Input: part model. Units: mm. Frame: model coordinates. A direction names the side the tool comes from. Coordinates: 2 decimals unless noted, no trailing zeros. Order: outer loops, then holes, each group sorted by start corner. A loop starts at its lowest first (then second) coordinate and runs counter-clockwise, first axis right, second up. Notation, with made-up numbers: (-22.5, 44.25) - (22.5, 44.25) arc R19 ccw to (22.5, 72.25) - close; hole circle Ø3 at (53.25, 61). An arc over 180 degrees is marked (long way). One line per question, with ' | ' between items.
from build123d import *

# Parameters (mm, degrees)
SKETCH1_R           = 2.75
SKETCH1_R_2         = 1.75
SKETCH1_W           = 5.5
SKETCH1_H           = 5.5
BOSS_EXTRUDE1_DEPTH = 1
SKETCH2_R           = 2.75
SKETCH2_R_2         = 1.75
BOSS_EXTRUDE2_DEPTH = 2.8
SKETCH3_W           = 25.5
SKETCH3_H           = 35.5
CUT_EXTRUDE1_DEPTH  = 2.8


with BuildPart() as part:
    # Sketch1 → Boss-Extrude1 (new body)
    # profile 1 of 11: a face of its own
    with BuildSketch(Plane(origin=(0, 0, 0), x_dir=(1, 0, 0), z_dir=(0, 1, 0))):
        with Locations((-15, -15)):
            Circle(SKETCH1_R)
        with Locations(Location((-15, -15, 0), (0, 0, 270))):
            Circle(SKETCH1_R_2, mode=Mode.SUBTRACT)
    # profile 2 of 11: a face of its own
    with BuildSketch(Plane(origin=(0, 0, 0), x_dir=(1, 0, 0), z_dir=(0, 1, 0))):
        with BuildLine():
            add(Edge.make_bspline(
                [(0, -7.5), (-1.590584075, -5.319747163), (-2.75, -2.75)],
                knots=[0.745921805, 0.745921805, 0.745921805, 1, 1, 1], degree=2))
            add(Edge.make_bspline(
                [(-15, -12.25), (-5.706246464, -10.868692238), (-2.75, -2.75)],
                knots=[0, 0, 0, 1, 1, 1], degree=2))
            ThreePointArc((-15, -12.25), (-13.055456352, -13.055456352), (-12.25, -15))
            ThreePointArc((-12.25, -15), (-12.459331286, -16.052379439), (-13.055456352, -16.944543648))
            add(Edge.make_bspline(
                [(-13.055456352, -16.944543648), (-4.669630712, -13.900778032), (0, -7.5)],
                knots=[0, 0, 0, 0.745921805, 0.745921805, 0.745921805], degree=2))
        make_face()
    # profile 3 of 11: a face of its own
    with BuildSketch(Plane(origin=(0, 0, 0), x_dir=(1, 0, 0), z_dir=(0, 1, 0))):
        with BuildLine():
            add(Edge.make_bspline(
                [(0, -7.5), (1.590584075, -5.319747163), (2.75, -2.75)],
                knots=[0.745921805, 0.745921805, 0.745921805, 1, 1, 1], degree=2))
            Line((2.75, -2.75), (-2.75, -2.75))
            add(Edge.make_bspline(
                [(0, -7.5), (-1.590584075, -5.319747163), (-2.75, -2.75)],
                knots=[0.745921805, 0.745921805, 0.745921805, 1, 1, 1], degree=2))
        make_face()
    # profile 4 of 11: a face of its own
    with BuildSketch(Plane(origin=(0, 0, 0), x_dir=(1, 0, 0), z_dir=(0, 1, 0))):
        Rectangle(SKETCH1_W, SKETCH1_H)
    # profile 5 of 11: a face of its own
    with BuildSketch(Plane(origin=(0, 0, 0), x_dir=(1, 0, 0), z_dir=(0, 1, 0))):
        with BuildLine():
            add(Edge.make_bspline(
                [(15, -12.25), (5.706246464, -10.868692238), (2.75, -2.75)],
                knots=[0, 0, 0, 1, 1, 1], degree=2))
            add(Edge.make_bspline(
                [(0, -7.5), (1.590584075, -5.319747163), (2.75, -2.75)],
                knots=[0.745921805, 0.745921805, 0.745921805, 1, 1, 1], degree=2))
            add(Edge.make_bspline(
                [(13.055456352, -16.944543648), (4.669630712, -13.900778032), (0, -7.5)],
                knots=[0, 0, 0, 0.745921805, 0.745921805, 0.745921805], degree=2))
            ThreePointArc((13.055456352, -16.944543648), (12.459331286, -13.947620561), (15, -12.25))
        make_face()
    # profile 6 of 11: a face of its own
    with BuildSketch(Plane(origin=(0, 0, 0), x_dir=(1, 0, 0), z_dir=(0, 1, 0))):
        with Locations((15, -15)):
            Circle(SKETCH1_R)
        with Locations(Location((15, -15, 0), (0, 0, 270))):
            Circle(SKETCH1_R_2, mode=Mode.SUBTRACT)
    # profile 7 of 11: a face of its own
    with BuildSketch(Plane(origin=(0, 0, 0), x_dir=(1, 0, 0), z_dir=(0, 1, 0))):
        with BuildLine():
            add(Edge.make_bspline(
                [(0, 7.5), (1.590584075, 5.319747163), (2.75, 2.75)],
                knots=[0.745921805, 0.745921805, 0.745921805, 1, 1, 1], degree=2))
            add(Edge.make_bspline(
                [(15, 12.25), (5.706246464, 10.868692238), (2.75, 2.75)],
                knots=[0, 0, 0, 1, 1, 1], degree=2))
            ThreePointArc((15, 12.25), (12.459331286, 13.947620561), (13.055456352, 16.944543648))
            add(Edge.make_bspline(
                [(13.055456352, 16.944543648), (4.669630712, 13.900778032), (0, 7.5)],
                knots=[0, 0, 0, 0.745921805, 0.745921805, 0.745921805], degree=2))
        make_face()
    # profile 8 of 11: a face of its own
    with BuildSketch(Plane(origin=(0, 0, 0), x_dir=(1, 0, 0), z_dir=(0, 1, 0))):
        with Locations((15, 15)):
            Circle(SKETCH1_R)
        with Locations(Location((15, 15, 0), (0, 0, 270))):
            Circle(SKETCH1_R_2, mode=Mode.SUBTRACT)
    # profile 9 of 11: a face of its own
    with BuildSketch(Plane(origin=(0, 0, 0), x_dir=(1, 0, 0), z_dir=(0, 1, 0))):
        with BuildLine():
            Line((-2.75, 2.75), (2.75, 2.75))
            add(Edge.make_bspline(
                [(0, 7.5), (1.590584075, 5.319747163), (2.75, 2.75)],
                knots=[0.745921805, 0.745921805, 0.745921805, 1, 1, 1], degree=2))
            add(Edge.make_bspline(
                [(0, 7.5), (-1.590584075, 5.319747163), (-2.75, 2.75)],
                knots=[0.745921805, 0.745921805, 0.745921805, 1, 1, 1], degree=2))
        make_face()
    # profile 10 of 11: a face of its own
    with BuildSketch(Plane(origin=(0, 0, 0), x_dir=(1, 0, 0), z_dir=(0, 1, 0))):
        with BuildLine():
            add(Edge.make_bspline(
                [(-15, 12.25), (-5.706246464, 10.868692238), (-2.75, 2.75)],
                knots=[0, 0, 0, 1, 1, 1], degree=2))
            add(Edge.make_bspline(
                [(0, 7.5), (-1.590584075, 5.319747163), (-2.75, 2.75)],
                knots=[0.745921805, 0.745921805, 0.745921805, 1, 1, 1], degree=2))
            add(Edge.make_bspline(
                [(-13.055456352, 16.944543648), (-4.669630712, 13.900778032), (0, 7.5)],
                knots=[0, 0, 0, 0.745921805, 0.745921805, 0.745921805], degree=2))
            ThreePointArc((-13.055456352, 16.944543648), (-12.459331286, 16.052379439), (-12.25, 15))
            ThreePointArc((-12.25, 15), (-13.055456352, 13.055456352), (-15, 12.25))
        make_face()
    # profile 11 of 11: a face of its own
    with BuildSketch(Plane(origin=(0, 0, 0), x_dir=(1, 0, 0), z_dir=(0, 1, 0))):
        with Locations((-15, 15)):
            Circle(SKETCH1_R)
        with Locations(Location((-15, 15, 0), (0, 0, 270))):
            Circle(SKETCH1_R_2, mode=Mode.SUBTRACT)
    extrude(amount=BOSS_EXTRUDE1_DEPTH)

    # Sketch2 → Boss-Extrude2 (add)
    # profile 1 of 4: a face of its own
    with BuildSketch(Plane(origin=(0, 1, 0), x_dir=(1, 0, 0), z_dir=(0, 1, 0))):
        with Locations(Location((-15, 15, 0), (0, 0, 270))):
            Circle(SKETCH2_R)
        with Locations(Location((-15, 15, 0), (0, 0, 270))):
            Circle(SKETCH2_R_2, mode=Mode.SUBTRACT)
    # profile 2 of 4: a face of its own
    with BuildSketch(Plane(origin=(0, 1, 0), x_dir=(1, 0, 0), z_dir=(0, 1, 0))):
        with Locations(Location((15, 15, 0), (0, 0, 270))):
            Circle(SKETCH2_R)
        with Locations(Location((15, 15, 0), (0, 0, 270))):
            Circle(SKETCH2_R_2, mode=Mode.SUBTRACT)
    # profile 3 of 4: a face of its own
    with BuildSketch(Plane(origin=(0, 1, 0), x_dir=(1, 0, 0), z_dir=(0, 1, 0))):
        with Locations(Location((15, -15, 0), (0, 0, 90))):
            Circle(SKETCH2_R)
        with Locations(Location((15, -15, 0), (0, 0, 270))):
            Circle(SKETCH2_R_2, mode=Mode.SUBTRACT)
    # profile 4 of 4: a face of its own
    with BuildSketch(Plane(origin=(0, 1, 0), x_dir=(1, 0, 0), z_dir=(0, 1, 0))):
        with Locations(Location((-15, -15, 0), (0, 0, 90))):
            Circle(SKETCH2_R)
        with Locations(Location((-15, -15, 0), (0, 0, 270))):
            Circle(SKETCH2_R_2, mode=Mode.SUBTRACT)
    extrude(amount=BOSS_EXTRUDE2_DEPTH)

    # Sketch3 → Cut-Extrude1 (cut)
    with BuildSketch(Plane(origin=(0, 3.8, 0), x_dir=(1, 0, 0), z_dir=(0, 1, 0))):
        Rectangle(SKETCH3_W, SKETCH3_H)
    extrude(amount=-CUT_EXTRUDE1_DEPTH, mode=Mode.SUBTRACT)


solid = part.part
Item 1: Ray query, line 1 (X direction, y = 2.7, z = 15); line 2 (Z direction, x = 16, y = 2.4); line 3 (Z direction, x = -13.5, y = 1.2). Return the intervals inside material, ascending.
Data:
line 1: -17.75 to -16.75, -13.25 to -12.75, 12.75 to 13.25, 16.75 to 17.75 | line 2: -17.56 to -16.44, -13.56 to -12.44, 12.44 to 13.56, 16.44 to 17.56 | line 3: -17.3 to -15.9, -14.1 to -12.7, 12.7 to 14.1, 15.9 to 17.3
Item 2: Access query for faces 5 (the face through (-17.75, 1.87, 14.9)), 6 (the face through (16.5, 1.9, -14.1)), 7 (the face through (12.75, 2, 15)). Directions: +Z, -Z, +X, -X, +Y, -Y. A direction counts if a zero-diameter tool reaches every point of the face in a straight line with its end or side. Return the directions, or none.
Data:
face 5: +Y | face 6: +Y, -Y | face 7: +Z, -Z, +Y
Item 3: Section B-B on z = -15. Count the separate pieces of the cut face and the enclosed holes in it, and give its area (3 significant figures).
Data:
separate pieces: 4 | enclosed holes: 0 | area: 19.5 mm^2
Item 4: Contact query for flat-ended pins moving along their axis: P1, Ø1.5, axis at y = 1.5, z = 2.5, coming from the -X side; P2, Ø0.5, axis at y = 0.5, z = 0.5, coming from the +X side; P3, Ø0.8, axis at y = 0.5, z = 0.5, coming from the -X side; P4, Ø1.4, axis at y = 2, z = -14.5, coming from the +X side. Output: stop coordinate, or through.
Data:
P1: x = -2.87 | P2: x = 2.75 | P3: x = -2.75 | P4: x = 17.75
Item 5: Section A-A on y = 2.15. Return the cut outline in (x, z), and give its area (3 significant figures).
Data:
outline: (-12.75, -16.58) - (-12.75, -13.42) arc R2.75 ccw (long way) to start; (-12.75, 13.42) - (-12.75, 16.58) arc R2.75 ccw (long way) to start; (12.75, -16.58) arc R2.75 ccw (long way) to (12.75, -13.42) - close; (12.75, 13.42) arc R2.75 ccw (long way) to (12.75, 16.58) - close; hole circle Ø3.5 at (-15, -15); hole circle Ø3.5 at (-15, 15); hole circle Ø3.5 at (15, -15); hole circle Ø3.5 at (15, 15) | area: 52.2 mm^2
Item 6: Draft query along X for faces 1 (the face through (2.75, 0.5, 0)), 2 (the face through (17.75, 1.87, -14.9)), 3 (the face through (-2.75, 0.5, 0)), 4 (the face through (-17, 3.8, -15)). Return one class per face: released by +X, released by -X, zero draft, split by the parting line, or undercut.
Data:
face 1: released by +X | face 2: undercut | face 3: released by -X | face 4: zero draft
